from build123d import *

# Parameters (mm, degrees)
SKETCH_1_R      = 15
EXTRUDE_1_DEPTH = 30
SKETCH_2_R      = 34
EXTRUDE_2_DEPTH = 5
CHAMFER_1_SIZE  = 2


with BuildPart() as part:
    # 草图1 → 凸台-拉伸1 (new body)
    with BuildSketch(Plane.XY):
        Circle(SKETCH_1_R)
    extrude(amount=EXTRUDE_1_DEPTH)

    # 草图2 → 凸台-拉伸2 (add)
    with BuildSketch(Plane.XY.offset(30)):
        Circle(SKETCH_2_R)
    extrude(amount=EXTRUDE_2_DEPTH)

    # 倒角1
    chamfer_1_edges = [part.edges().sort_by_distance(p)[0] for p in [
        (-15, 0, 0),
    ]]
    chamfer(chamfer_1_edges, length=CHAMFER_1_SIZE)


solid = part.part
Build history of the part. All positions in model axes, mm. A direction names the side the tool comes from. Coordinates: 2 decimals unless noted, no trailing zeros. Write each loop counter-clockwise with the first axis right and the second up, starting at its lowest first coordinate (ties: lowest second). Pieces come first, ordered by that corner, then holes.
(1) Drill centre lines: line 1 (Z direction, x = 4.5, y = 18.5); line 2 (X direction, y = 9.5, z = 33.5); line 3 (Y direction, x = 8, z = 31). Where is each one in solid material? Low to high.
(2) Pin check, flat tips, straight feed: pin 1 Ø1.5 at (x, y) = (-14.5, -18) entering from -Z; pin 2 Ø8 at (y, z) = (7.5, 11.5) entering from +X; pin 3 Ø12 at (x, z) = (-11, 29.5) entering from -Y. Stop position of each tip, or through.
(3) Cut at C-C on z = 33. List the corners of the cut face in (x, y).
(4) 3-axis set-ups, long thin cutter, end or side, ignore diameter. For faces 1 (the flat face through (15, -7, 30)), 2 (the flat face through (0, 0, 35)): which of +Z, -Z, +X, -X, +Y, -Y reach the whole face in a straight line?
(5) Cut at A-A on x = 0. List the corners of the cut face in (y, z), and give its area (3 significant figures).
(6) Cut at D-D on z = 26. List the corners of the cut face in (x, y).
Working result:
1. line 1: z = 30 to 35
1. line 2: x = -32.65 to 32.65
1. line 3: y = -33.05 to 33.05
2. pin 1: stops at z = 30
2. pin 2: stops at x = 14.59
2. pin 3: stops at y = -33.63
3. outline: circle Ø68 at (0, 0)
4. face 1: -Z
4. face 2: +Z, +X, -X, +Y, -Y
5. outline: (-34, 30) - (-15, 30) - (-15, 2) - (-13, 0) - (13, 0) - (15, 2) - (15, 30) - (34, 30) - (34, 35) - (-34, 35) - close
5. area: 1,240 mm2
6. outline: circle Ø30 at (0, 0)
